Build history of the part. All positions in model axes, mm. Give positions to 0.01 mm unless a question says otherwise; leave off trailing zeros. Order: outer loops, then holes, each group sorted by start corner. A loop starts at its lowest first (then second) coordinate and runs counter-clockwise, first axis right, second up. Notation, with made-up numbers: M 79,-34.5 L 134,-34.5 A12 cw 134,-28.5 Z; hole C 1,-17 d6. An arc over 180 degrees is marked long. Answer as CSV lines item,"result".
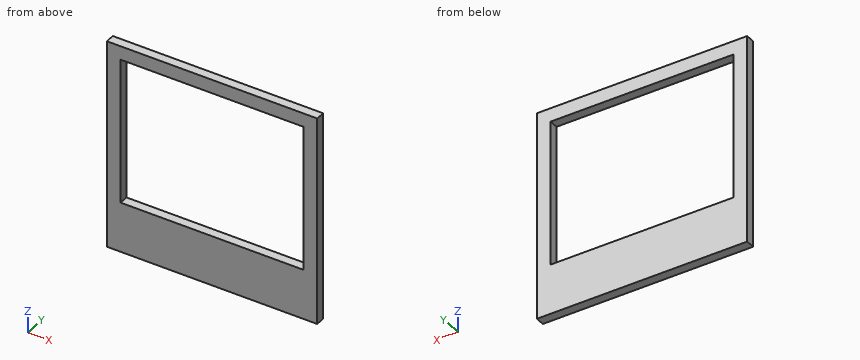
from build123d import *

# Parameters (mm, degrees)
F0_W     = 230
F0_H     = 40
F0_H_2   = 190
F0_W_2   = 200
F0_H_3   = 159.9997122972
F1_DEPTH = 10


# Not quite as in the source:
# - a feature names something its author has since deleted; it is built from what else it names


with BuildPart() as f1:
    # F0 (on Front) → F1 (new body)
    with BuildSketch(Plane.XZ):
        with Locations((0.0107780099, -35.0002877028)):
            Rectangle(F0_W, F0_H)
        with Locations((0.0107780099, 79.9997122972)):
            Rectangle(F0_W, F0_H_2)
        with Locations((0.0107780099, 79.9998561486)):
            Rectangle(F0_W_2, F0_H_3, mode=Mode.SUBTRACT)
    extrude(amount=F1_DEPTH)


solid = f1.part
Item 1: Band-saw the part on A-A (x = -97). Give the cut face in (y, z), and give its area (3 significant figures).
Geometry says:
outline,"M -10,-55 L 0,-55 L 0,0 L -10,0 Z; M -10,160 L 0,160 L 0,175 L -10,175 Z"
area,"700 mm2"
Item 2: Band-saw the part on B-B (z = 82). Give the cut face in (x, y), and give its area (3 significant figures).
Geometry says:
outline,"M -114.99,-10 L -99.99,-10 L -99.99,0 L -114.99,0 Z; M 100.01,-10 L 115.01,-10 L 115.01,0 L 100.01,0 Z"
area,"300 mm2"
Item 3: Band-saw the part on C-C (y = -3). Give the cut face in (x, z).
Geometry says:
outline,"M -114.99,-55 L 115.01,-55 L 115.01,175 L -114.99,175 Z; hole M -99.99,0 L 100.01,0 L 100.01,160 L -99.99,160 Z"
Item 4: Probe line 1 along Z through (x, y) = (54.5, -1.75); line 2 along X through (y, z) = (-9.25, 158). List the from-to ranges inside material, lowest first. Write a range as from..to.
Geometry says:
line 1,"z = -55..0, 160..175"
line 2,"x = -114.99..-99.99, 100.01..115.01"
